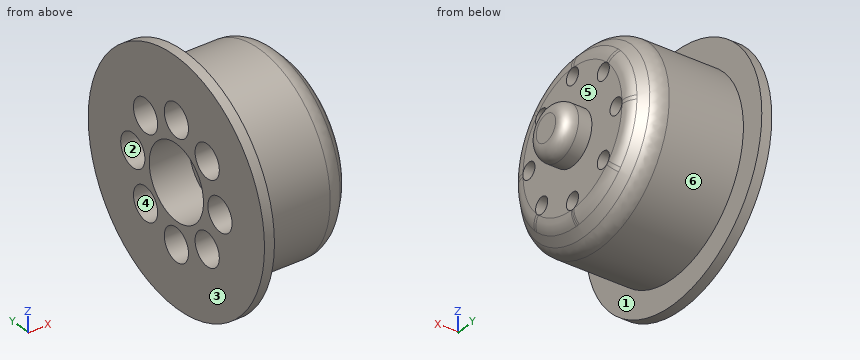
from build123d import *

# Parameters (mm, degrees)
FILLET1_R          = 2
SKETCH4_R          = 5.6
CUT_EXTRUDE3_DEPTH = 6
SKETCH5_R          = 1.25
CUT_EXTRUDE4_DEPTH = 16.75
SKETCH6_R          = 2.5
CUT_EXTRUDE5_DEPTH = 11.75
FILLET2_R          = 3


with BuildPart() as part:
    # Sketch1 → Revolve1 (revolve)
    with BuildSketch(Plane(origin=(0, 0, 0), x_dir=(1, 0, 0), z_dir=(0, 1, 0))):
        Polygon((-4.630434783, 14.4), (7.869565217, 14.4), (10.619565217, 11.390476118), (10.619565217, 4), (14.619565217, 4), (14.619565217, 0), (13.372742768, 0), (-6.130434783, 0), (-6.130434783, 18.2), (-4.630434783, 18.2), align=None)
    revolve(axis=Axis((-12.391304348, 0, 0), (1, 0, 0)))

    # Fillet1
    fillet1_edges = [part.edges().sort_by_distance(p)[0] for p in [
        (14.619565217, 0, 4),
    ]]
    fillet(fillet1_edges, radius=FILLET1_R)

    # Sketch4 → Cut-Extrude3 (cut)
    with BuildSketch(Plane.ZY.offset(6.130434783)):
        Circle(SKETCH4_R)
    extrude(amount=-CUT_EXTRUDE3_DEPTH, mode=Mode.SUBTRACT)

    # Sketch5 → Cut-Extrude4 (cut)
    with BuildSketch(Plane(origin=(10.619565217, 0, 0), x_dir=(0, 0, -1), z_dir=(1, 0, 0))):
        with Locations((0, 9)):
            Circle(SKETCH5_R)
        with Locations((6.363961031, 6.363961031)):
            Circle(SKETCH5_R)
        with Locations((9, 0)):
            Circle(SKETCH5_R)
        with Locations((6.363961031, -6.363961031)):
            Circle(SKETCH5_R)
        with Locations((0, -9)):
            Circle(SKETCH5_R)
        with Locations((-6.363961031, -6.363961031)):
            Circle(SKETCH5_R)
        with Locations((-9, 0)):
            Circle(SKETCH5_R)
        with Locations((-6.363961031, 6.363961031)):
            Circle(SKETCH5_R)
    extrude(amount=-CUT_EXTRUDE4_DEPTH, mode=Mode.SUBTRACT)

    # Sketch6 → Cut-Extrude5 (cut)
    with BuildSketch(Plane.ZY.offset(6.130434783)):
        with Locations((0, 9)):
            Circle(SKETCH6_R)
        with Locations((6.363961031, 6.363961031)):
            Circle(SKETCH6_R)
        with Locations((9, 0)):
            Circle(SKETCH6_R)
        with Locations((6.363961031, -6.363961031)):
            Circle(SKETCH6_R)
        with Locations((0, -9)):
            Circle(SKETCH6_R)
        with Locations((-6.363961031, -6.363961031)):
            Circle(SKETCH6_R)
        with Locations((-9, 0)):
            Circle(SKETCH6_R)
        with Locations((-6.363961031, 6.363961031)):
            Circle(SKETCH6_R)
    extrude(amount=-CUT_EXTRUDE5_DEPTH, mode=Mode.SUBTRACT)

    # Fillet2
    fillet2_edges = [part.edges().sort_by_distance(p)[0] for p in [
        (7.869565217, 0, 14.4),
        (10.619565217, 0, 11.390476118),
    ]]
    fillet(fillet2_edges, radius=FILLET2_R)


solid = part.part
Read the model definition and answer for the solid it produces. Units are mm, in the model's axes. Face numbers are marked on the shaded views. A direction names the side the tool comes from. Round coordinates to 2 decimals unless told otherwise and drop trailing zeros. Write each loop counter-clockwise with the first axis right and the second up, starting at its lowest first coordinate (ties: lowest second). Pieces come first, ordered by that corner, then holes.
1. Given pin 1 Ø1.5 at (y, z) = (-3, 14) entering from +X; pin 2 Ø6 at (y, z) = (6.36, -6.36) entering from +X; pin 3 Ø4 at (y, z) = (-6.36, 6.36) entering from -X, each flat-ended and moving along its own axis, determine where each tip first touches the part or whether it passes through.
2. The part is cut by section D-D, the plane z = -15.5. Determine the outline of the cut face in (x, y), then the cut area to 3 significant figures.
3. The part is cut by section A-A, the plane x = 2.25. State how many separate pieces and enclosed holes the cut face has, then the cut area to 3 significant figures.
4. Determine the mould class of the marked faces 4, 5 and 6 for opening direction Y: pulls with the +Y half, pulls with the -Y half, needs draft (parallel to the pull), parting line crosses it, or undercut.
5. Which of the six approach directions +Z, -Z, +X, -X, +Y, -Y give full straight-line access (tool end or side, diameter ignored) to the marked faces 1, 2 and 3?
6. Straight lines are drawn through the part: L1, parallel to Y at x = 0.5, z = 0; L2, parallel to Y at x = -3.1, z = 0; L3, parallel to Y at x = -4.5, z = 6. For each, find the intervals that lie inside material, in ascending order.
7. The part is cut by section C-C, the plane z = 16.5. Determine the outline of the cut face in (x, y).
Values:
1. pin 1: stops at x = 8.62
1. pin 2: stops at x = 10.62
1. pin 3: stops at x = 5.62
2. outline: (-6.13, -9.54) - (-4.63, -9.54) - (-4.63, 9.54) - (-6.13, 9.54) - close
2. area: 28.6 mm2
3. separate pieces: 1
3. enclosed holes: 8
3. area: 494 mm2
4. face 4: undercut
4. face 5: needs draft
4. face 6: parting line crosses it
5. face 1: +X
5. face 2: -X
5. face 3: +Z, -Z, -X, +Y, -Y
6. L1: y = -14.4 to -11.5, -6.5 to 6.5, 11.5 to 14.4
6. L2: y = -14.4 to -11.5, -6.5 to -5.6, 5.6 to 6.5, 11.5 to 14.4
6. L3: y = -13.09 to -8.84, -3.89 to 3.89, 8.84 to 13.09
7. outline: (-6.13, -7.68) - (-4.63, -7.68) - (-4.63, 7.68) - (-6.13, 7.68) - close
